Work out the finished part from the listing and answer in its coordinate system (mm). Round coordinates to 2 decimals unless told otherwise and drop trailing zeros. Write each loop counter-clockwise with the first axis right and the second up, starting at its lowest first coordinate (ties: lowest second). Pieces come first, ordered by that corner, then holes. Notation, with made-up numbers: (59, 18) -> (109, 18) arc R3 ccw to (109, 22) -> close; hole circle Ø9 at (43, 36). An arc over 180 degrees is marked (long way). One line per item, written item: value.
```python
from build123d import *

# Parameters (mm, degrees)
SKETCH_1_R          = 5.5
EXTRUDE_1_DEPTH     = 5
SCALE_1_SCALE       = 0.3
SKETCH_3_W          = 17.210108286
SKETCH_3_H          = 5.437935386
CUT_EXTRUDE_2_DEPTH = 20
FILLET_1_R          = 4
FILLET_2_R          = 1
SKETCH_4_W          = 94.817377104
SKETCH_4_H          = 9.548741528
CUT_EXTRUDE_3_DEPTH = 20
FILLET_3_R          = 1


with BuildPart() as part:
    # 草图1 → 凸台-拉伸1 (new body)
    with BuildSketch(Plane.XY):
        with BuildLine():
            Line((0, 10), (500, 10))
            ThreePointArc((500, 10), (510, 0), (500, -10))
            Line((500, -10), (0, -10))
            ThreePointArc((0, -10), (-10, 0), (0, 10))
        make_face()
        Circle(SKETCH_1_R, mode=Mode.SUBTRACT)
        with Locations((500, 0)):
            Circle(SKETCH_1_R, mode=Mode.SUBTRACT)
    extrude(amount=EXTRUDE_1_DEPTH)


with BuildPart() as part_1:
    # 缩放比例1: scaled about (0, 0, 0)
    add(part.part.scale(SCALE_1_SCALE))

    # 草图3 → 切除-拉伸2 (cut)
    with BuildSketch(Plane.XY.offset(1.5)):
        with Locations((13.002886653, -2.718967693)):
            Rectangle(SKETCH_3_W, SKETCH_3_H)
        with Locations((136.997113347, -2.718967693)):
            Rectangle(SKETCH_3_W, SKETCH_3_H)
    extrude(amount=-CUT_EXTRUDE_2_DEPTH, mode=Mode.SUBTRACT)

    # 圆角1
    # the kernel refuses this fillet: 4 mm, written as the material it takes off along each edge
    with BuildSketch(Plane(origin=(145.60216749, -3, 11.182458366), x_dir=(1, 0, 0), z_dir=(0, 0, -1))) as fillet_1_piece_1:
        with BuildLine():
            CenterArc((3.872983346, -4), FILLET_1_R, 90, 75.522487814)
            Line((0, -3), (-0.077459667, -2.98))
            ThreePointArc((-0.077459667, -2.98), (-0.08, -1.5), (-0.08, 0))
            Line((-0.08, 0), (0, 0.08))
            Line((0, 0.08), (3.872983346, 0.08))
            Line((3.872983346, 0.08), (3.872983346, 0))
        make_face()
    extrude(amount=20.864916731, mode=Mode.SUBTRACT)
    with BuildSketch(Plane(origin=(4.39783251, -3, 11.182458366), x_dir=(-1, 0, 0), z_dir=(0, 0, -1))) as fillet_1_piece_2:
        with BuildLine():
            CenterArc((3.872983346, 4), FILLET_1_R, 194.477512186, 75.522487814)
            Line((0, 3), (-0.077459667, 2.98))
            ThreePointArc((-0.077459667, 2.98), (-0.08, 1.5), (-0.08, 0))
            Line((-0.08, 0), (0, -0.08))
            Line((0, -0.08), (3.872983346, -0.08))
            Line((3.872983346, -0.08), (3.872983346, 0))
        make_face()
    extrude(amount=20.864916731, mode=Mode.SUBTRACT)

    # 圆角2
    fillet_2_edges = [part_1.edges().sort_by_distance(p)[0] for p in [
        (128.392059204, -3, 0.75),
        (21.607940796, -3, 0.75),
        (21.607940796, 0, 0.75),
        (128.392059204, 0, 0.75),
    ]]
    fillet(fillet_2_edges, radius=FILLET_2_R)

    # 草图4 → 切除-拉伸3 (cut)
    with BuildSketch(Plane.XY.offset(1.5)):
        with Locations((74.821866685, 4.774370764)):
            Rectangle(SKETCH_4_W, SKETCH_4_H)
    extrude(amount=-CUT_EXTRUDE_3_DEPTH, mode=Mode.SUBTRACT)

    # 圆角3
    fillet_3_edges = [part_1.edges().sort_by_distance(p)[0] for p in [
        (122.230555237, 3, 0.75),
        (27.413178133, 3, 0.75),
        (122.230555237, 0, 0.75),
        (27.413178133, 0, 0.75),
    ]]
    fillet(fillet_3_edges, radius=FILLET_3_R)


solid = part_1.part
```
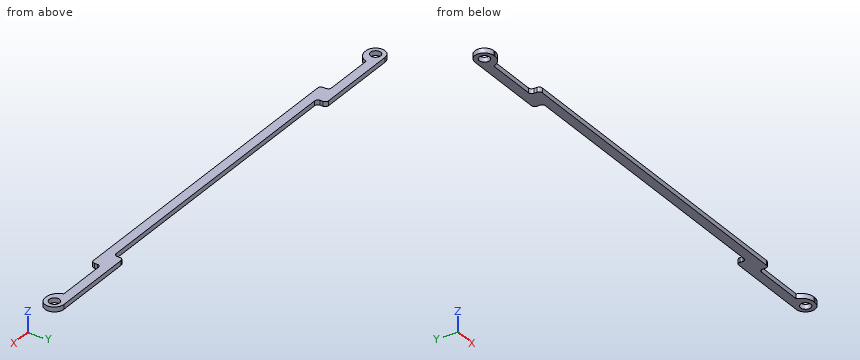
(1) Consider probe 1 along Y at (x, z) = (0, 0.75); probe 2 along X at (y, z) = (1, 0.65); probe 3 along X at (y, z) = (0.5, 0.15). Determine where each line is inside the solid, lowest interval first.
Reported:
probe 1: y = -3 to -1.65, 1.65 to 3
probe 2: x = -2.83 to -1.31, 1.31 to 27.41, 122.23 to 148.69, 151.31 to 152.83
probe 3: x = -2.96 to -1.57, 1.57 to 27.55, 122.1 to 148.43, 151.57 to 152.96
(2) Find section B-B on x = 87. Give the vertices of the cut face in (y, z), plus the area to 3 significant figures.
Reported:
outline: (-3, 0) -> (0, 0) -> (0, 1.5) -> (-3, 1.5) -> close
area: 4.50 mm2
(3) Flat-ended cylindrical pins translate along their axes: pin 1 Ø0.5 at (y, z) = (-1.5, 0.5) entering from +X; pin 2 Ø0.5 at (y, z) = (1.5, 1) entering from -X; pin 3 Ø3 at (x, y) = (150, 0) entering from -Z. Find the tip coordinate at first contact, or state that the pin passes through.
Reported:
pin 1: stops at x = 152.73
pin 2: stops at x = -2.73
pin 3: passes through
(4) Find section A-A on z = 1.05. Give the vertices of the cut face in (x, y), plus the area to 3 significant figures.
Reported:
outline: (0, -3) -> (0.52, -3) arc R4 ccw to (4.4, 0) -> (20.61, 0) arc R1 cw to (21.61, -1) -> (21.61, -2) arc R1 ccw to (22.61, -3) -> (127.39, -3) arc R1 ccw to (128.39, -2) -> (128.39, -1) arc R1 cw to (129.39, 0) -> (145.6, 0) arc R4 ccw to (149.48, -3) -> (150, -3) arc R3 ccw to (150, 3) -> (123.23, 3) arc R1 ccw to (122.23, 2) -> (122.23, 1) arc R1 cw to (121.23, 0) -> (28.41, 0) arc R1 cw to (27.41, 1) -> (27.41, 2) arc R1 ccw to (26.41, 3) -> (0, 3) arc R3 ccw to start; hole circle Ø3.3 at (0, 0); hole circle Ø3.3 at (150, 0)
area: 517 mm2
